Could you check a few things on this model? Use its own coordinates, in mm. A direction names the side the tool comes from. Round coordinates to 2 decimals unless told otherwise and drop trailing zeros. Loops run counter-clockwise (first coordinate to the right, second up) from the corner with the lowest first, then second, coordinate; pieces in that order, holes last. Notation, with made-up numbers: (-32, 21.5) -> (-27, 21.5) arc R16 ccw to (-27, 40.5) -> close; hole circle Ø7 at (-18.5, 57.5). An arc over 180 degrees is marked (long way). Put each result on its own line as item: value. Start each with the question number.
1. I'm going to push flat-ended pins straight in: P1, Ø1.5, axis at x = -6, z = -3.5, coming from the -Y side; P2, Ø6, axis at x = -21, z = -5, coming from the +Y side; P3, Ø5, axis at x = 10.5, z = -4, coming from the -Y side. Where does each tip first touch, or does it pass through?
2. Which directions (+Z, -Z, +X, -X, +Y, -Y) give clear straight access to the entire face, cutting with the end or side of a thin tool? Please do faces 1 (the flat face through (-30.125, 2, -2)), 2 (the cylindrical face through (-28, 0, -5)).
3. Imagine slicing it at A-A, the plane y = 0. Please give me the cut outline in (x, z) (3 decimals), and give its area (4 significant figures).
4. I need wall thicknesses on line 1 (Y direction, x = -26.25, z = 0); line 2 (X direction, y = -6.5, z = -0.5) (3 decimals); line 3 (X direction, y = -6, z = 2.75) (3 decimals). Which ranges of each line are inside material? Lowest first, please. Write a range as [from, to].
5. Imagine slicing it at C-C, the plane x = 4.5. Please give me the cut outline in (y, z), and give its area (3 significant figures).
6. Imagine slicing it at D-D, the plane z = -5.75. Count the separate pieces of the cut face and the enclosed holes in it, and give its area (3 significant figures).
```python
from build123d import *


with BuildPart() as part:
    # Esboço1 → Revolução1 (revolve)
    with BuildSketch(Plane.XY, mode=Mode.PRIVATE) as revolu_o1_sk:
        Polygon((-15.245, 0), (-15.245, 2.5), (-30.125, 2.5), (-30.125, 5), (-25.125, 5), (-25.125, 7.5), (-23.955, 5.7), (-22.785, 7.5), (-21.615, 5.7), (-20.445, 7.5), (-19.275, 5.7), (-18.105, 7.5), (-16.935, 5.7), (-15.765, 7.5), (30.125, 7.5), (30.125, 0), align=None)
    revolve(revolu_o1_sk.sketch.rotate(Axis((0, 0, 0), (1, 0, 0)), 90), axis=Axis((0, 0, 0), (1, 0, 0)))


solid = part.part
```
Entries:
1. P1: y = -6.98
1. P2: y = 7.21
1. P3: y = -7.35
2. face 1: +Z, -Z, -X, +Y, -Y
2. face 2: -X
3. outline: (-30.125, -5) -> (-25.125, -5) -> (-25.125, -7.5) -> (-23.955, -5.7) -> (-22.785, -7.5) -> (-21.615, -5.7) -> (-20.445, -7.5) -> (-19.275, -5.7) -> (-18.105, -7.5) -> (-16.935, -5.7) -> (-15.765, -7.5) -> (30.125, -7.5) -> (30.125, 7.5) -> (-15.765, 7.5) -> (-16.935, 5.7) -> (-18.105, 7.5) -> (-19.275, 5.7) -> (-20.445, 7.5) -> (-21.615, 5.7) -> (-22.785, 7.5) -> (-23.955, 5.7) -> (-25.125, 7.5) -> (-25.125, 5) -> (-30.125, 5) -> (-30.125, 2.5) -> (-15.245, 2.5) -> (-15.245, -2.5) -> (-30.125, -2.5) -> close
3. area: 787.5 mm^2
4. line 1: [-5, -2.5], [2.5, 5]
4. line 2: [-25.125, -24.487], [-23.423, -22.147], [-21.083, -19.807], [-18.743, -17.467], [-16.403, 30.125]
4. line 3: [-25.125, -24.54], [-23.37, -22.2], [-21.03, -19.86], [-18.69, -17.52], [-16.35, 30.125]
5. outline: circle Ø15 at (0, 0)
5. area: 177 mm^2
6. separate pieces: 5
6. enclosed holes: 0
6. area: 499 mm^2
